Part print with two shaded views. Sizes in mm from the minimum x, y, z corner. Coordinates: 2 decimals unless noted, no trailing zeros. Order: outer loops, then holes, each group sorted by start corner. A loop starts at its lowest first (then second) coordinate and runs counter-clockwise, first axis right, second up.
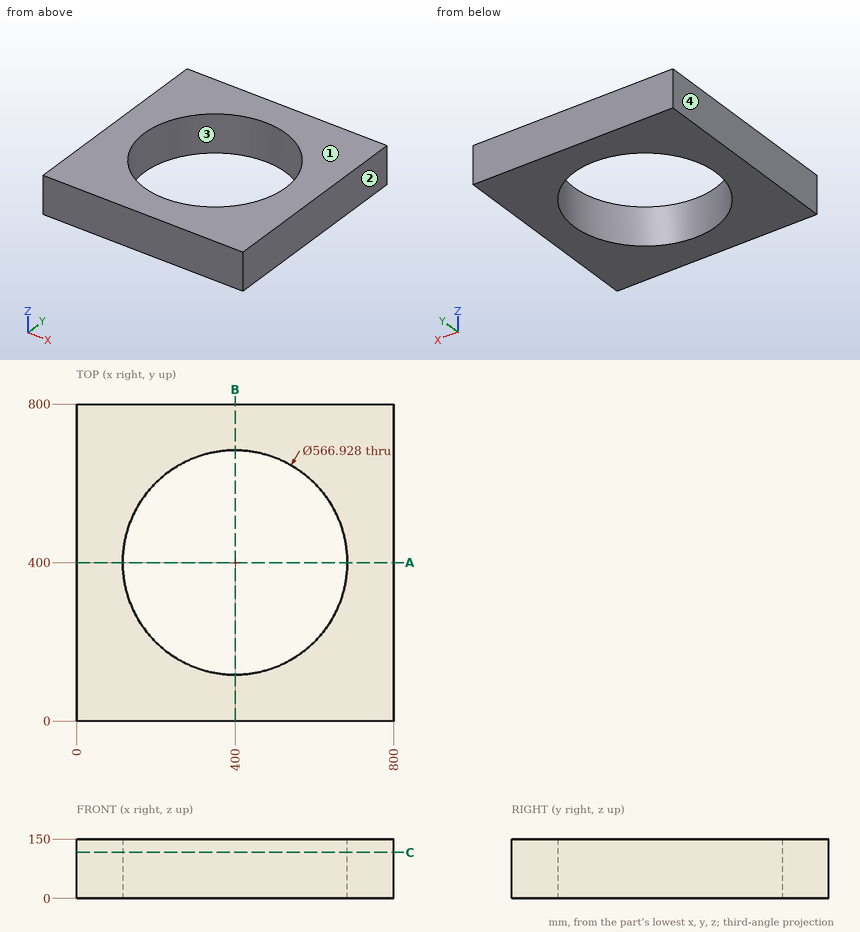
Q1. Pin check, flat tip, straight feed: pin 1 Ø10 at (x, z) = (352, 53.5) entering from -Y. Stop position of the tip, or through.
Results list:
pin 1: stops at y = 0
Q2. Mould opens along X. For the marked faces 1, 2, 3 and 4 say: pulls with the +X half, pulls with the -X half, needs draft (parallel to the pull), parting line crosses it, or undercut.
Results list:
face 1: needs draft
face 2: pulls with the +X half
face 3: undercut
face 4: pulls with the -X half
Q3. Wall check: line 1 along Y through (x, z) = (400, 45.5); line 2 along Y through (x, z) = (628.5, 142.5). Give the ranges that are in metal, low to high.
Results list:
line 1: y = 0 to 116.54, 683.46 to 800
line 2: y = 0 to 232.25, 567.75 to 800
Q4. Cut at A-A on y = 400. Write the cut outline in (x, z), and give its area (3 significant figures).
Results list:
outline: (0, 0) - (116.54, 0) - (116.54, 150) - (0, 150) - close; (683.46, 0) - (800, 0) - (800, 150) - (683.46, 150) - close
area: 35,000 mm2
Q5. Cut at C-C on z = 116. Write the cut outline in (x, y), and give its area (3 significant figures).
Results list:
outline: (0, 0) - (800, 0) - (800, 800) - (0, 800) - close; hole circle Ø566.93 at (400, 400)
area: 388,000 mm2
